from build123d import *

# Parameters (mm, degrees)
F0_W     = 357.378
F0_H     = 357.378
F1_DEPTH = 51.562
F2_T     = -0.762
F4_D     = 3.2639
F4_DEPTH = 0.762
F4_TIP   = 0.9805744872
F6_D     = 3.2639


with BuildPart() as f1:
    # F0 (on Top) → F1 (new body)
    with BuildSketch(Plane.XY):
        Rectangle(F0_W, F0_H)
    extrude(amount=F1_DEPTH)

    # F2
    f2_openings = [f1.faces().sort_by_distance(p)[0] for p in [
        (0, 0, 51.562),
    ]]
    offset(amount=F2_T, openings=f2_openings)

    # F4
    with Locations(Plane.XZ.offset(178.689)):
        with Locations((139.7, 7.112), (0, 7.112), (-139.7, 7.112)):
            Hole(F4_D / 2, depth=F4_DEPTH)
            with Locations((0, 0, -(F4_DEPTH + F4_TIP / 2))):  # 118° drill point
                Cone(0, F4_D / 2, F4_TIP, mode=Mode.SUBTRACT)

    # F6 (through all)
    with Locations(Plane(origin=(-178.689, 0, 0), x_dir=(0, -1, 0), z_dir=(-1, 0, 0))):
        with Locations((-139.7, 7.112), (0, 7.112), (139.7, 7.112)):
            Hole(F6_D / 2)


solid = f1.part
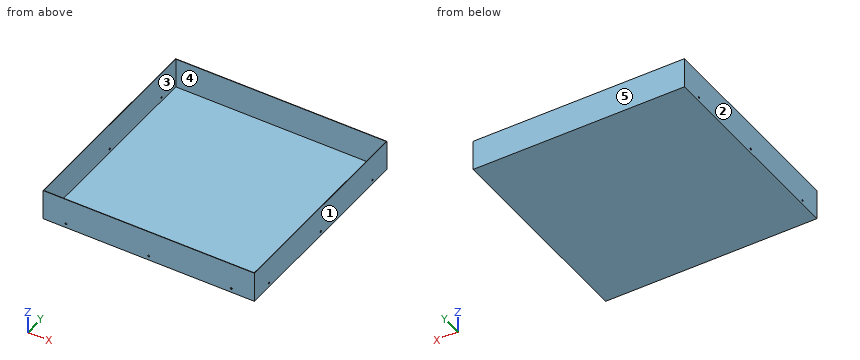
Verification items for the finished model (mm, model axes). Face numbers are marked on the shaded views. A direction names the side the tool comes from. Coordinates: 2 decimals unless noted, no trailing zeros. Write each loop counter-clockwise with the first axis right and the second up, starting at its lowest first coordinate (ties: lowest second). Pieces come first, ordered by that corner, then holes. Notation, with made-up numbers: (71, -25.75) - (119, -25.75) arc R20 ccw to (119, -3.75) - close; hole circle Ø5 at (-15.75, -1.75). An arc over 180 degrees is marked (long way). Answer as a JSON object with one key per item and string values.
(1) Gauge pin test, flat ends, axial feed: pin 1 Ø6 at (x, y) = (-61.5, 111) entering from +Z; pin 2 Ø2.5 at (x, z) = (0, 7.112) entering from -Y. Record the tip position at first contact, or that the pin passes through.
Report:
{"pin 1": "z = 0.76", "pin 2": "y = 177.93"}
(2) Thickness scan on line 1 along X through (y, z) = (17.5, 19.5); line 2 along Z through (x, y) = (-178.45, 0). Record the ranges inside material, lowest first.
Report:
{"line 1": "-178.69 to -177.93, 177.93 to 178.69", "line 2": "0 to 5.48, 8.74 to 51.56"}
(3) Cross-section at A-A on z = 19. Record the cut outline in (x, y), plus the area to 3 significant figures.
Report:
{"outline": "(-178.69, -178.69) - (178.69, -178.69) - (178.69, 178.69) - (-178.69, 178.69) - close; hole (-177.93, -177.93) - (177.93, -177.93) - (177.93, 177.93) - (-177.93, 177.93) - close", "area": "1,090 mm^2"}
(4) Tool access check on the marked faces 4 and 5. Record the directions out of +Z, -Z, +X, -X, +Y, -Y that give a thin tool (end or side, any length) a straight path to the whole face; none if there is none.
Report:
{"face 4": "+Z", "face 5": "+Z, -Z, +X, -X, +Y"}
(5) Mould release check, pull along X, two halves, no side actions. Record for the marked faces 1, 2 and 3: pulls with the +X half, pulls with the -X half, needs draft (parallel to the pull), parting line crosses it, or undercut.
Report:
{"face 1": "pulls with the +X half", "face 2": "pulls with the -X half", "face 3": "undercut"}
(6) Cross-section at B-B on y = 10. Record the cut outline in (x, z), plus the area to 3 significant figures.
Report:
{"outline": "(-178.69, 0) - (178.69, 0) - (178.69, 51.56) - (177.93, 51.56) - (177.93, 0.76) - (-177.93, 0.76) - (-177.93, 51.56) - (-178.69, 51.56) - close", "area": "350 mm^2"}
